Read the model definition and answer for the solid it produces. Units are mm, in the model's axes. Coordinates: 2 decimals unless noted, no trailing zeros. Order: outer loops, then holes, each group sorted by start corner. A loop starts at its lowest first (then second) coordinate and runs counter-clockwise, first axis right, second up. Notation, with made-up numbers: (5.5, 35.5) -> (54.5, 35.5) arc R9 cw to (54.5, 46.5) -> close; hole circle Ø10 at (68, 50.5). An arc over 180 degrees is marked (long way). Return JSON: item names as keys, results as strings. Group by question number.
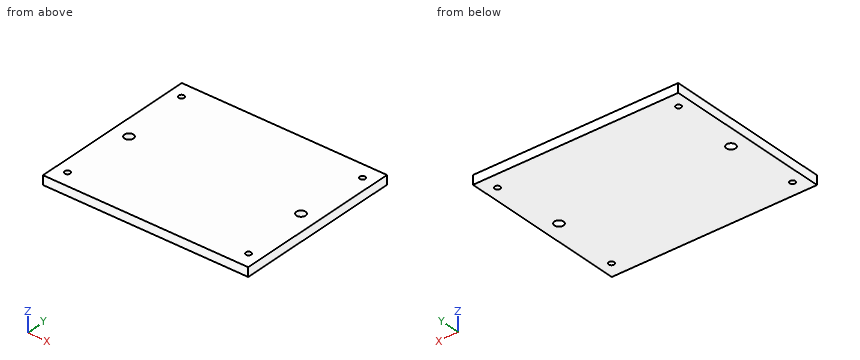
```python
from build123d import *

# Parameters (mm, degrees)
F0_W     = 340
F0_H     = 280
F1_DEPTH = 15
F3_D     = 9
F4_D     = 15


with BuildPart() as f1:
    # F0 (on Top) → F1 (new body)
    with BuildSketch(Plane.XY):
        Rectangle(F0_W, F0_H)
    extrude(amount=F1_DEPTH)

    # F3 (through all)
    with Locations(Plane.XY.offset(15)):
        with Locations((-150, 115), (-150, -115), (150, -115), (150, 115)):
            Hole(F3_D / 2)

    # F4 (through all)
    with Locations(Plane.XY.offset(15)):
        with Locations((142.5, 0), (-142.5, 0)):
            Hole(F4_D / 2)


solid = f1.part
```
1. Find section B-B on y = 0. Determine the outline of the cut face in (x, z).
2. Find section A-A on y = 115. Determine the outline of the cut face in (x, z), and give its area (3 significant figures).
3. Given pin 1 (11.5 mm diameter, centred on x = -150, y = 115, fed in from +Z), flat-ended and moving along its own axis, determine where the tip first touches the part or whether it passes through.
4. Straight lines are drawn through the part: L1, parallel to Y at x = 142, z = 6.5; L2, parallel to Y at x = -144, z = 10.5. For each, find the intervals that lie inside material, in ascending order.
Result:
{
 "1": {"outline": "(-170, 0) -> (-150, 0) -> (-150, 15) -> (-170, 15) -> close; (-135, 0) -> (135, 0) -> (135, 15) -> (-135, 15) -> close; (150, 0) -> (170, 0) -> (170, 15) -> (150, 15) -> close"},
 "2": {"outline": "(-170, 0) -> (-154.5, 0) -> (-154.5, 15) -> (-170, 15) -> close; (-145.5, 0) -> (145.5, 0) -> (145.5, 15) -> (-145.5, 15) -> close; (154.5, 0) -> (170, 0) -> (170, 15) -> (154.5, 15) -> close", "area": "4,830 mm^2"},
 "3": {"pin 1": "z = 15"},
 "4": {"L1": "-140 to -7.48, 7.48 to 140", "L2": "-140 to -7.35, 7.35 to 140"}
}
